from build123d import *

# Parameters (mm, degrees)
MODEL_R                 = 1.60291439
MODEL_R_2               = 2.755009107
MODEL_W                 = 5.5
MODEL_H                 = 5
MODEL_H_2               = 5.009107468
SALIENTE_EXTRUIR1_DEPTH = 3


with BuildPart() as part:
    # Model → Saliente-Extruir1 (new body)
    with BuildSketch(Plane.XY):
        with BuildLine():
            Line((146.331612735, 52.084906554), (71.693408409, 52.084905051))
            ThreePointArc((71.693408409, 52.084905051), (71.339211023, 52.231618412), (71.192497662, 52.585815798))
            Line((71.192497662, 52.585815798), (71.192497662, 58.093853412))
            ThreePointArc((71.192497662, 58.093853412), (70.605644218, 59.510642955), (69.188854675, 60.097496399))
            Line((69.188854675, 60.097496399), (64.864840233, 60.097496399))
            ThreePointArc((64.864840233, 60.097496399), (64.422309224, 59.831272426), (64.45017085, 59.315585867))
            ThreePointArc((64.45017085, 59.315585867), (61.174282726, 53.138492666), (57.898394601, 59.315585867))
            ThreePointArc((57.898394601, 59.315585867), (57.926256228, 59.831272427), (57.483725218, 60.097496399))
            Line((57.483725218, 60.097496399), (53.159710777, 60.097496399))
            ThreePointArc((53.159710777, 60.097496399), (51.742921234, 59.510642955), (51.15606779, 58.093853412))
            Line((51.15606779, 58.093853412), (51.15606779, 52.585818804))
            ThreePointArc((51.15606779, 52.585818804), (51.009354429, 52.231621418), (50.655157043, 52.084908057))
            Line((50.655157043, 52.084908057), (20.928604766, 52.084908057))
            Line((20.928604766, 52.084908057), (15.919497298, 52.084908057))
            ThreePointArc((15.919497298, 52.084908057), (12.37752344, 50.617774447), (10.91038983, 47.075800589))
            Line((10.91038983, 47.075800589), (10.91038983, 12.625568804))
            ThreePointArc((10.91038983, 12.625568804), (12.377524274, 9.083594111), (15.919499658, 7.616461335))
            Line((15.919499658, 7.616461335), (35.219821515, 7.616461335))
            ThreePointArc((35.219821515, 7.616461335), (35.81301385, 7.810960614), (36.17587477, 8.318936073))
            Line((36.17587477, 8.318936073), (37.739622557, 13.313231589))
            ThreePointArc((37.739622557, 13.313231589), (38.102483477, 13.821207048), (38.695675812, 14.015706326))
            Line((38.695675812, 14.015706326), (146.331612735, 14.013271547))
            Line((146.331612735, 14.013271547), (253.967549659, 14.015706326))
            ThreePointArc((253.967549659, 14.015706326), (254.560741993, 13.821207048), (254.923602913, 13.313231589))
            Line((254.923602913, 13.313231589), (256.487350701, 8.318936073))
            ThreePointArc((256.487350701, 8.318936073), (256.85021162, 7.810960614), (257.443403955, 7.616461335))
            Line((257.443403955, 7.616461335), (276.743725812, 7.616461335))
            ThreePointArc((276.743725812, 7.616461335), (280.285701196, 9.083594111), (281.75283564, 12.625568804))
            Line((281.75283564, 12.625568804), (281.75283564, 47.075800589))
            ThreePointArc((281.75283564, 47.075800589), (280.285702031, 50.617774447), (276.743728172, 52.084908057))
            Line((276.743728172, 52.084908057), (271.734620704, 52.084908057))
            Line((271.734620704, 52.084908057), (242.008068427, 52.084908057))
            ThreePointArc((242.008068427, 52.084908057), (241.653871041, 52.231621418), (241.50715768, 52.585818804))
            Line((241.50715768, 52.585818804), (241.50715768, 58.093853412))
            ThreePointArc((241.50715768, 58.093853412), (240.920304237, 59.510642955), (239.503514693, 60.097496399))
            Line((239.503514693, 60.097496399), (235.179500252, 60.097496399))
            ThreePointArc((235.179500252, 60.097496399), (234.736969242, 59.831272427), (234.764830869, 59.315585867))
            ThreePointArc((234.764830869, 59.315585867), (231.488942744, 53.138492666), (228.21305462, 59.315585867))
            ThreePointArc((228.21305462, 59.315585867), (228.240916247, 59.831272426), (227.798385238, 60.097496399))
            Line((227.798385238, 60.097496399), (223.474370795, 60.097496399))
            ThreePointArc((223.474370795, 60.097496399), (222.057581252, 59.510642955), (221.470727808, 58.093853412))
            Line((221.470727808, 58.093853412), (221.470727808, 52.585815798))
            ThreePointArc((221.470727808, 52.585815798), (221.324014447, 52.231618412), (220.969817061, 52.084905051))
            Line((220.969817061, 52.084905051), (146.331612735, 52.084906554))
        make_face()
        with Locations((61.174282726, 43.070186654)):
            Circle(MODEL_R, mode=Mode.SUBTRACT)
        with Locations((231.488942744, 43.070186654)):
            Circle(MODEL_R, mode=Mode.SUBTRACT)
        with Locations((153.845273937, 33.04908905)):
            Circle(MODEL_R, mode=Mode.SUBTRACT)
        with Locations((33.011476123, 24.647426727)):
            Circle(MODEL_R_2, mode=Mode.SUBTRACT)
        with Locations((259.651749347, 24.647426727)):
            Circle(MODEL_R_2, mode=Mode.SUBTRACT)
        with Locations((153.84026483, 40.558196518)):
            Rectangle(MODEL_W, MODEL_H, mode=Mode.SUBTRACT)
        with Locations((153.84026483, 25.535427848)):
            Rectangle(MODEL_W, MODEL_H_2, mode=Mode.SUBTRACT)
    extrude(amount=SALIENTE_EXTRUIR1_DEPTH)


solid = part.part
Geometry: final body of the model. Coordinates: model frame, mm. Coordinates: 2 decimals unless noted, no trailing zeros. Order: outer loops, then holes, each group sorted by start corner. A loop starts at its lowest first (then second) coordinate and runs counter-clockwise, first axis right, second up.
(1) Section query B-B (z = 1.7). State how many separate pieces and enclosed holes the cut face has, plus the area to 3 significant figures.
(2) First-contact query: pin 1 (0.9 mm diameter, centred on x = 152.5, z = 1, fed in from -Y); pin 2 (4 mm diameter, centred on x = 179.5, y = 37.5, fed in from -Z); pin 3 (0.9 mm diameter, centred on x = 27, z = 2, fed in from +Y). Flat tips, straight axial feed; report the tip coordinate or a pass-through.
(3) Section query A-A (x = 75). Return the cut outline in (y, z), plus the area to 3 significant figures.
(4) Material intervals for probe 1 along X at (y, z) = (24, 1.2); probe 2 along Y at (x, z) = (188.5, 1.95); probe 3 along Y at (x, z) = (30, 2.85), sorted ascending.
(5) Draft query along X for faces 1 (the face through (144, 34, 3)), 2 (the face through (12.34, 9.12, 1.48)), 3 (the face through (257.465, 22.971, 1.479)), 4 (the face through (35.64, 25.47, 1.48)). Return one class per face: pulls with the +X half, pulls with the -X half, needs draft (parallel to the pull), parting line crosses it, or undercut.
Solution:
1. separate pieces: 1
1. enclosed holes: 7
1. area: 10,700 mm2
2. pin 1: stops at y = 14.01
2. pin 2: stops at z = 0
2. pin 3: stops at y = 52.08
3. outline: (14.01, 0) - (52.08, 0) - (52.08, 3) - (14.01, 3) - close
3. area: 114 mm2
4. probe 1: x = 10.91 to 30.33, 35.69 to 151.09, 156.59 to 256.97, 262.33 to 281.75
4. probe 2: y = 14.01 to 52.08
4. probe 3: y = 7.62 to 52.08
5. face 1: needs draft
5. face 2: pulls with the -X half
5. face 3: undercut
5. face 4: undercut
